```python
from build123d import *

# Parameters (mm, degrees)
SKETCH1_W           = 20
SKETCH1_H           = 40
BOSS_EXTRUDE1_DEPTH = 151
SKETCH2_W           = 80
SKETCH2_H           = 80
BOSS_EXTRUDE2_DEPTH = 5
SKETCH3_R           = 2.5
CUT_EXTRUDE1_DEPTH  = 166.939748102
CUT_EXTRUDE2_REACH  = 167.94
SKETCH4_R           = 2.15


with BuildPart() as part:
    # Sketch1 → Boss-Extrude1 (new body)
    with BuildSketch(Plane(origin=(0, 0, 0), x_dir=(1, 0, 0), z_dir=(0, 1, 0))):
        Rectangle(SKETCH1_W, SKETCH1_H)
    extrude(amount=BOSS_EXTRUDE1_DEPTH)

    # Sketch2 → Boss-Extrude2 (add)
    with BuildSketch(Plane(origin=(0, 151, 0), x_dir=(1, 0, 0), z_dir=(0, 1, 0))):
        Rectangle(SKETCH2_W, SKETCH2_H)
    extrude(amount=BOSS_EXTRUDE2_DEPTH)

    # Sketch3 → Cut-Extrude1 (cut, through all)
    with BuildSketch(Plane(origin=(0, 156, 0), x_dir=(1, 0, 0), z_dir=(0, 1, 0))):
        with Locations(Location((0, 10, 0), (0, 0, 270))):
            Circle(SKETCH3_R)
        with Locations(Location((0, -10, 0), (0, 0, 270))):
            Circle(SKETCH3_R)
    extrude(amount=-CUT_EXTRUDE1_DEPTH, mode=Mode.SUBTRACT)

    # Sketch4 → Cut-Extrude2 (cut, up to next)
    with BuildSketch(Plane(origin=(0, 156, 0), x_dir=(1, 0, 0), z_dir=(0, 1, 0)), mode=Mode.PRIVATE) as cut_extrude2_sk1:
        with Locations(Location((-22, 31, 0), (0, 0, 270))):
            Circle(SKETCH4_R)
    cut_extrude2_tool1 = extrude(cut_extrude2_sk1.sketch, amount=-CUT_EXTRUDE2_REACH, mode=Mode.PRIVATE) & part.part
    # Sketch4 → Cut-Extrude2 (cut, up to next)
    with BuildSketch(Plane(origin=(0, 156, 0), x_dir=(1, 0, 0), z_dir=(0, 1, 0)), mode=Mode.PRIVATE) as cut_extrude2_sk2:
        with Locations(Location((27, 27, 0), (0, 0, 270))):
            Circle(SKETCH4_R)
    cut_extrude2_tool2 = extrude(cut_extrude2_sk2.sketch, amount=-CUT_EXTRUDE2_REACH, mode=Mode.PRIVATE) & part.part
    # Sketch4 → Cut-Extrude2 (cut, up to next)
    with BuildSketch(Plane(origin=(0, 156, 0), x_dir=(1, 0, 0), z_dir=(0, 1, 0)), mode=Mode.PRIVATE) as cut_extrude2_sk3:
        with Locations(Location((-27, -27, 0), (0, 0, 270))):
            Circle(SKETCH4_R)
    cut_extrude2_tool3 = extrude(cut_extrude2_sk3.sketch, amount=-CUT_EXTRUDE2_REACH, mode=Mode.PRIVATE) & part.part
    # Sketch4 → Cut-Extrude2 (cut, up to next)
    with BuildSketch(Plane(origin=(0, 156, 0), x_dir=(1, 0, 0), z_dir=(0, 1, 0)), mode=Mode.PRIVATE) as cut_extrude2_sk4:
        with Locations(Location((27, -27, 0), (0, 0, 270))):
            Circle(SKETCH4_R)
    cut_extrude2_tool4 = extrude(cut_extrude2_sk4.sketch, amount=-CUT_EXTRUDE2_REACH, mode=Mode.PRIVATE) & part.part
    add(cut_extrude2_tool1.solids().sort_by_distance((-22, 156, -31))[0], mode=Mode.SUBTRACT)
    add(cut_extrude2_tool2.solids().sort_by_distance((27, 156, -27))[0], mode=Mode.SUBTRACT)
    add(cut_extrude2_tool3.solids().sort_by_distance((-27, 156, 27))[0], mode=Mode.SUBTRACT)
    add(cut_extrude2_tool4.solids().sort_by_distance((27, 156, 27))[0], mode=Mode.SUBTRACT)


solid = part.part
```
The model under review builds one solid part; all positions refer to its coordinate system, in mm. A direction names the side the tool comes from. Round coordinates to 2 decimals unless told otherwise and drop trailing zeros. Loops run counter-clockwise (first coordinate to the right, second up) from the corner with the lowest first, then second, coordinate; pieces in that order, holes last. Notation, with made-up numbers: M 84.5,83.25 L 98.5,83.25 A14 ccw 98.5,105.25 Z; hole C -15.5,15 d8. An arc over 180 degrees is marked long. Put each result on its own line as item: value.
Q1. Consider section C-C, the plane x = -27. Give the boundary of the cut face in (y, z), then the cut area to 4 significant figures.
Result set:
outline: M 151,-40 L 156,-40 L 156,24.85 L 151,24.85 Z; M 151,29.15 L 156,29.15 L 156,40 L 151,40 Z
area: 378.5 mm²
Q2. For pin 1 (1.5 mm diameter, centred on y = 81, z = 4.5, fed in from +X); pin 2 (2.5 mm diameter, centred on x = -22, z = -31, fed in from -Y); pin 3 (7 mm diameter, centred on x = 27, z = 27, fed in from -Y); pin 4 (8 mm diameter, centred on y = 57, z = -5.5, fed in from -X), all flat-tipped, find the tip position at first contact; note any pin that passes through.
Result set:
pin 1: stops at x = 10
pin 2: passes through
pin 3: stops at y = 151
pin 4: stops at x = -10
Q3. Consider section A-A, the plane x = 27. Give the boundary of the cut face in (y, z).
Result set:
outline: M 151,-40 L 156,-40 L 156,-29.15 L 151,-29.15 Z; M 151,-24.85 L 156,-24.85 L 156,24.85 L 151,24.85 Z; M 151,29.15 L 156,29.15 L 156,40 L 151,40 Z
Q4. Consider section B-B, the plane z = -10. Give the boundary of the cut face in (x, y), then the cut area to 3 significant figures.
Result set:
outline: M -40,151 L -10,151 L -10,0 L -2.5,0 L -2.5,156 L -40,156 Z; M 2.5,0 L 10,0 L 10,151 L 40,151 L 40,156 L 2.5,156 Z
area: 2,640 mm²
Q5. Machinability: for faces 5 (the flat face through (10, 74, 0)), 6 (the flat face through (0, 74, -20)), 7 (the cylindrical face through (0.1, 79.1, 7.5)), which of the approach directions +Z, -Z, +X, -X, +Y, -Y give a long, thin tool a straight path to every point of the face, cutting with its end or side? Answer none if there is none.
Result set:
face 5: +Z, -Z, +X, -Y
face 6: -Z, +X, -X, -Y
face 7: +Y, -Y
Q6. To check wall thickness, follow L1, parallel to X at y = 152, z = 27; L2, parallel to X at y = 114, z = 10; L3, parallel to X at y = 87.5, z = 18.5. State the ranges of each line that lie inside material, in increasing order.
Result set:
L1: x = -40 to -29.15, -24.85 to 24.85, 29.15 to 40
L2: x = -10 to -2.5, 2.5 to 10
L3: x = -10 to 10
Q7. Mouldability with a two-part tool opening along Z and no side actions: class faces 1 (the flat face through (0, 74, 20)), 2 (the flat face through (-1, 153, -40)), 3 (the cylindrical face through (27.65, 153.54, -24.95)), 4 (the flat face through (-10, 74, 0)) as released by +Z, released by -Z, zero draft, split by the parting line, or undercut.
Result set:
face 1: released by +Z
face 2: released by -Z
face 3: undercut
face 4: zero draft
Q8. Consider section D-D, the plane z = 27. Give the boundary of the cut face in (x, y).
Result set:
outline: M -40,151 L -29.15,151 L -29.15,156 L -40,156 Z; M -24.85,151 L 24.85,151 L 24.85,156 L -24.85,156 Z; M 29.15,151 L 40,151 L 40,156 L 29.15,156 Z
